Check sheet for the drawn part. Datum: minimum x, y, z corner. Units: mm. A direction names the side the tool comes from. Give positions to 0.01 mm unless a question says otherwise; leave off trailing zeros. Order: outer loops, then holes, each group sorted by start corner. A loop starts at its lowest first (then second) coordinate and runs counter-clockwise, first axis right, second up.
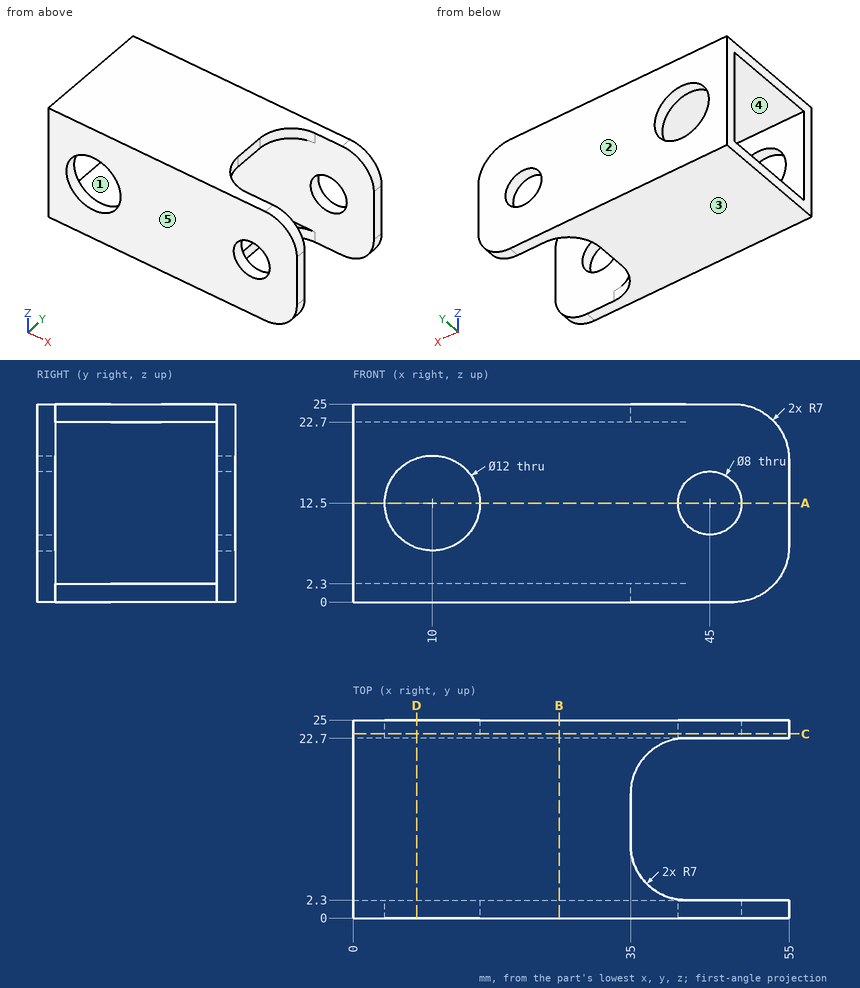
Item 1: Sectioned sample at A-A (z = 12.5). Enter the section's corners in (x, y).
Reported:
outline: (0, 0) - (4, 0) - (4, 2.3) - (0, 2.3) - close; (0, 22.7) - (4, 22.7) - (4, 25) - (0, 25) - close; (16, 0) - (41, 0) - (41, 2.3) - (16, 2.3) - close; (16, 22.7) - (41, 22.7) - (41, 25) - (16, 25) - close; (49, 0) - (55, 0) - (55, 2.3) - (49, 2.3) - close; (49, 22.7) - (55, 22.7) - (55, 25) - (49, 25) - close
Item 2: Sectioned sample at B-B (x = 26). Enter the section's corners in (y, z).
Reported:
outline: (0, 0) - (25, 0) - (25, 25) - (0, 25) - close; hole (2.3, 2.3) - (22.7, 2.3) - (22.7, 22.7) - (2.3, 22.7) - close
Item 3: Sectioned sample at C-C (y = 23.25). Enter the section's corners in (x, z).
Reported:
outline: (0, 0) - (48, 0) arc R7 ccw to (55, 7) - (55, 18) arc R7 ccw to (48, 25) - (0, 25) - close; hole circle Ø12 at (10, 12.5); hole circle Ø8 at (45, 12.5)
Item 4: Set-up check for the marked faces 1 and 2: record each of +Z, -Z, +X, -X, +Y, -Y from which the full face is reachable in a straight line by a thin tool's end or side.
Reported:
face 1: +X, -X
face 2: +Z, -Z, +X, -X, +Y
Item 5: Gauge pin test, flat ends, axial feed: pin 1 (7.5 mm diameter, centred on x = 14.5, z = 8.5, fed in from -Y); pin 2 (2.5 mm diameter, centred on y = 13.5, z = 24, fed in from +X). Record the tip position at first contact, or that the pin passes through.
Reported:
pin 1: stops at y = 0
pin 2: stops at x = 35
Item 6: Scan lines: L1, parallel to X at y = 23.65, z = 12.5; L2, parallel to Y at x = 35, z = 11.25. Record each from-to range of solid material in increasing order.
Reported:
L1: x = 0 to 4, 16 to 41, 49 to 55
L2: y = 0 to 2.3, 22.7 to 25
Item 7: Sectioned sample at D-D (x = 8). Enter the section's corners in (y, z), and give its area (3 significant figures).
Reported:
outline: (0, 0) - (25, 0) - (25, 6.84) - (22.7, 6.84) - (22.7, 2.3) - (2.3, 2.3) - (2.3, 6.84) - (0, 6.84) - close; (0, 18.16) - (2.3, 18.16) - (2.3, 22.7) - (22.7, 22.7) - (22.7, 18.16) - (25, 18.16) - (25, 25) - (0, 25) - close
area: 157 mm2
Item 8: Draft check along Z on the marked faces 3, 4 and 5. Enter one of: released by +Z, released by -Z, zero draft, split by the parting line, or undercut.
Reported:
face 3: released by -Z
face 4: undercut
face 5: zero draft
